from build123d import *

# Parameters (mm, degrees)
F0_W          = 53.2894550107
F0_H          = 50
F0_W_2        = 43.2894550107
F0_H_2        = 40
F1_DEPTH      = 25
F3_ANGLE_BACK = 90
F3_ANGLE      = 180


with BuildPart() as f1:
    # F0 (on Front) → F1 (new body)
    with BuildSketch(Plane.XZ):
        with Locations((-26.6447275054, 25)):
            Rectangle(F0_W, F0_H)
        with Locations((-26.6447275054, 25)):
            Rectangle(F0_W_2, F0_H_2, mode=Mode.SUBTRACT)
    extrude(amount=F1_DEPTH)

    # F2 (on face) → F3 (revolve)
    with BuildSketch(Plane.XZ.offset(25), mode=Mode.PRIVATE) as f3_sk:
        with BuildLine():
            ThreePointArc((0, 0), (17.6776695297, 7.3223304703), (25, 25))
            ThreePointArc((25, 25), (17.6776695297, 42.6776695297), (0, 50))
            Line((0, 50), (0, 45))
            ThreePointArc((0, 45), (14.1421356237, 39.1421356237), (20, 25))
            ThreePointArc((20, 25), (14.1421356237, 10.8578643763), (0, 5))
            Line((0, 5), (0, 0))
        make_face()
    revolve(f3_sk.sketch.rotate(Axis((0, -25, 25), (0, 0, -1)), -F3_ANGLE_BACK), axis=Axis((0, -25, 25), (0, 0, -1)), revolution_arc=F3_ANGLE)

    # F2 (on face) → F5 section 0
    with BuildSketch(Plane.XZ.offset(25)):
        Polygon((-53.2894550107, 44.7783708427), (-53.2894550107, 50), (-112.8771346405, 0), (-53.2894550107, 0), (-53.2894550107, 4), (-101.8872249626, 4), align=None)
    # F4 (on face) → F5 section 1
    with BuildSketch(Plane(origin=(0, 0, 0), x_dir=(-1, 0, 0), z_dir=(0, 1, 0))):
        Polygon((160.5148010362, 0), (53.2894550107, 50), (53.2894550107, 45.5864883242), (142.4719670216, 4), (53.2894550107, 4), (53.2894550107, 0), align=None)
    loft()


solid = f1.part
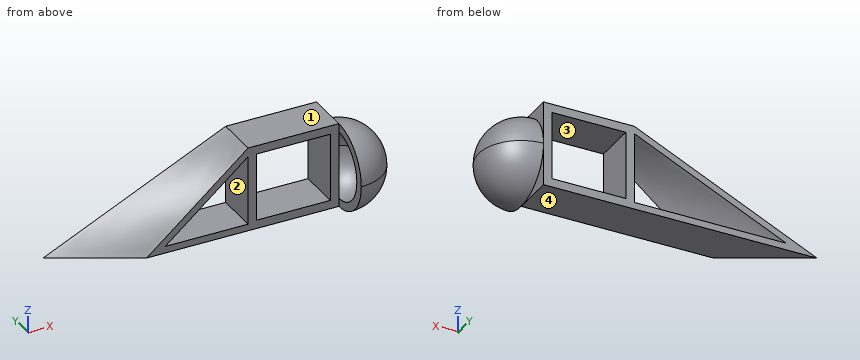
Input: part model. Units: mm. Frame: model coordinates. Face numbers are marked on the shaded views. Coordinates: 2 decimals unless noted, no trailing zeros. Loops run counter-clockwise (first coordinate to the right, second up) from the corner with the lowest first, then second, coordinate; pieces in that order, holes last.
Q1. Cut plane C-C (y = -35). Output: boundary loops of the cut face in (x, z), then the cut area to 3 significant figures.
Q2. Material intervals for line 1 (Z direction, x = -11, y = -7); line 2 (X direction, y = -12, z = 13); line 3 (X direction, y = -21.5, z = 21.5), sorted ascending.
Q3. Cut plane A-A (x = -15.5). Output: boundary loops of the cut face in (y, z).
Q4. Draft query along Z for the marked faces 1, 2, 3 and 4. Return one class per face: +Z half, -Z half, draft (parallel to the pull), parting line (faces both ways), or undercut.
Q5. Contact query for flat-ended pins moving along their axis: pin 1 (12.5 mm diameter, centred on y = -14.5, z = 21, fed in from -X); pin 2 (20 mm diameter, centred on y = -8.5, z = 33.5, fed in from -X); pin 3 (25 mm diameter, centred on x = -69, z = 17.5, fed in from -Y); pin 4 (12 mm diameter, centred on x = -57.5, y = -32.5, fed in from +Z). Output: stop coordinate, or through.
Q6. Cut plane B-B (z = 7). Give the number of separate pieces and of enclosed holes in the cut face, then the cut area to 3 significant figures.
Working result:
1. outline: (0, 2.09) arc R22.91 ccw to (0, 47.91) - (0, 42.32) arc R17.32 cw to (0, 7.68) - close
1. area: 353 mm2
2. line 1: z = 0 to 5, 45 to 50
2. line 2: x = -115.72 to -107.76, -53.29 to -48.29, -5 to 0, 9.33 to 17.66
2. line 3: x = -91.06 to -84.34, -53.29 to -48.29, -5 to 0, 19.38 to 24.51
3. outline: (-25, 0) - (0, 0) - (0, 5) - (-25, 5) - close; (-25, 45) - (0, 45) - (0, 50) - (-25, 50) - close
4. face 1: +Z half
4. face 2: undercut
4. face 3: undercut
4. face 4: -Z half
5. pin 1: stops at x = -112.27
5. pin 2: stops at x = -103.95
5. pin 3: stops at y = -25
5. pin 4: passes through
6. separate pieces: 3
6. enclosed holes: 0
6. area: 800 mm2
